Design review of the part shown in the three views and the two pictorial views. Dimensions are in mm from the part's minimum x, y and z. Coordinates: 2 decimals unless noted, no trailing zeros. Write each loop counter-clockwise with the first axis right and the second up, starting at its lowest first coordinate (ties: lowest second). Pieces come first, ordered by that corner, then holes.
Q1. For pin 1 Ø1 at (x, y) = (57.5, 1) entering from +Z; pin 2 Ø0.6 at (y, z) = (1, 16) entering from +X; pin 3 Ø1 at (y, z) = (1, 19) entering from -X; pin 4 Ø6 at (x, z) = (57, 16.5) entering from +Y, all flat-tipped, find the tip position at first contact; note any pin that passes through.
Q2. Take a section at C-C, the plane z = 2. Write out the cut boundary in (x, y) (3 decimals), plus the area to 3 significant figures.
Q3. Take a section at A-A, the plane z = 18.25. Write out the cut boundary in (x, y) (3 decimals).
Q4. Take a section at B-B, the plane y = 1.55. Write out the cut boundary in (x, z).
Q5. For L1, parallel to X at y = 1.75, z = 16.5; L2, parallel to X at y = 0.4, z = 21.25; L3, parallel to Z at x = 43, y = 1.65, list the stretches that pass through material, from the lowest coordinate up.
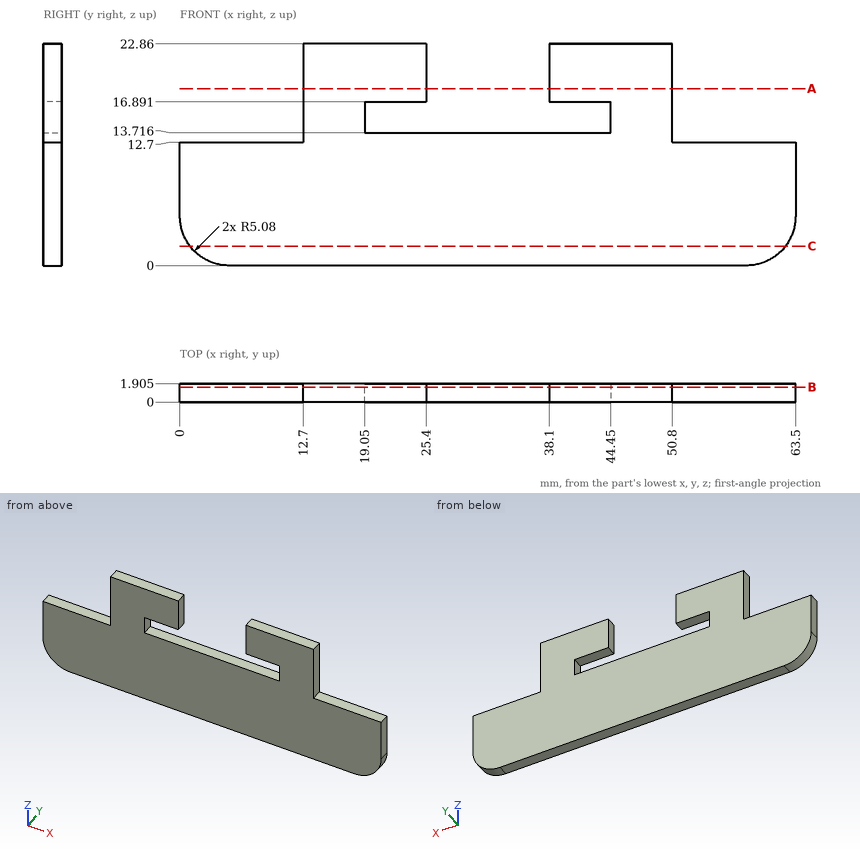
Responses:
1. pin 1: stops at z = 12.7
1. pin 2: stops at x = 50.8
1. pin 3: stops at x = 12.7
1. pin 4: passes through
2. outline: (1.04, 0) - (62.46, 0) - (62.46, 1.905) - (1.04, 1.905) - close
2. area: 117 mm2
3. outline: (12.7, 0) - (25.4, 0) - (25.4, 1.905) - (12.7, 1.905) - close; (38.1, 0) - (50.8, 0) - (50.8, 1.905) - (38.1, 1.905) - close
4. outline: (0, 5.08) arc R5.08 ccw to (5.08, 0) - (58.42, 0) arc R5.08 ccw to (63.5, 5.08) - (63.5, 12.7) - (50.8, 12.7) - (50.8, 22.86) - (38.1, 22.86) - (38.1, 16.89) - (44.45, 16.89) - (44.45, 13.72) - (19.05, 13.72) - (19.05, 16.89) - (25.4, 16.89) - (25.4, 22.86) - (12.7, 22.86) - (12.7, 12.7) - (0, 12.7) - close
5. L1: x = 12.7 to 19.05, 44.45 to 50.8
5. L2: x = 12.7 to 25.4, 38.1 to 50.8
5. L3: z = 0 to 13.72, 16.89 to 22.86
